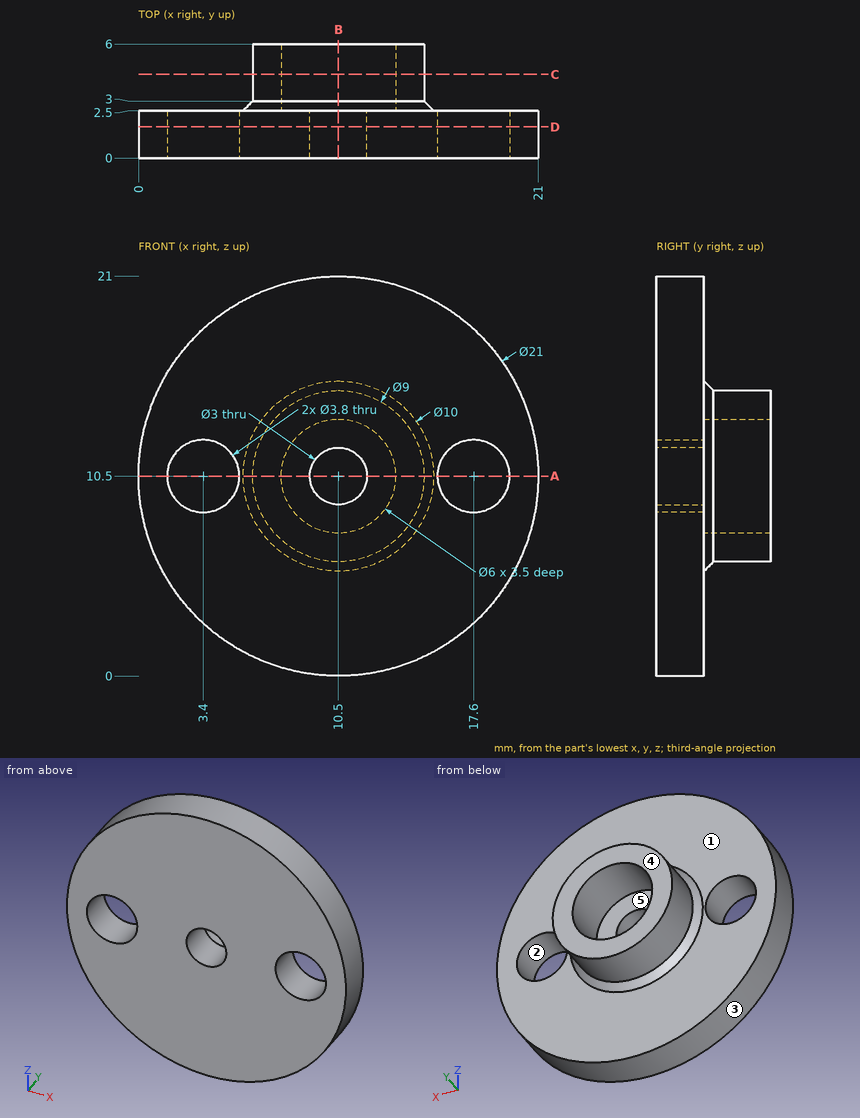
Verification items for this drawing (mm, ordinates from the low corner). A direction names the side the tool comes from. Round coordinates to 2 decimals unless told otherwise and drop trailing zeros. Loops run counter-clockwise (first coordinate to the right, second up) from the corner with the lowest first, then second, coordinate; pieces in that order, holes last. Notation, with made-up numbers: (80.25, 88) - (89.25, 88) arc R24 cw to (89.25, 102) - close; hole circle Ø5 at (-36.75, 2.25). An arc over 180 degrees is marked (long way). Write item = value, one per line.
Q1. Sectioned sample at D-D on y = 1.65. Record the boundary of the cut face in (x, z), plus the area to 3 significant figures.
Here are the results:
outline = circle Ø21 at (10.5, 10.5); hole circle Ø3.8 at (3.4, 10.5); hole circle Ø3 at (10.5, 10.5); hole circle Ø3.8 at (17.6, 10.5)
area = 317 mm^2
Q2. Depth check by flat-ended pin: pin 1 (3 mm diameter, centred on x = 17.6, z = 10.5, fed in from +Y); pin 2 (1.8 mm diameter, centred on x = 10, z = 12, fed in from +Y); pin 3 (1 mm diameter, centred on y = 5, z = 6, fed in from -X); pin 4 (1.5 mm diameter, centred on y = 2.5, z = 12, fed in from +X). Enter the tip coordinate at first touch or a pass-through.
Here are the results:
pin_1 = through
pin_2 = 2.5
pin_3 = 8.44
pin_4 = 20.97
Q3. Sectioned sample at B-B on x = 10.5. Record the boundary of the cut face in (y, z).
Here are the results:
outline = (0, 0) - (2.5, 0) - (2.5, 5.5) - (3, 6) - (6, 6) - (6, 7.5) - (2.5, 7.5) - (2.5, 9) - (0, 9) - close; (0, 12) - (2.5, 12) - (2.5, 13.5) - (6, 13.5) - (6, 15) - (3, 15) - (2.5, 15.5) - (2.5, 21) - (0, 21) - close
Q4. Mould release check, pull along Z, two halves, no side actions. Record for the marked faces 1, 2 and 3: +Z half, -Z half, draft (parallel to the pull), parting line (faces both ways), or undercut.
Here are the results:
face_1 = draft
face_2 = undercut
face_3 = parting line
Q5. Tool access check on the marked faces 4 and 5. Record the directions out of +Z, -Z, +X, -X, +Y, -Y that give a thin tool (end or side, any length) a straight path to the whole face; none if there is none.
Here are the results:
face_4 = +Z, -Z, +X, -X, +Y
face_5 = +Y
Q6. Sectioned sample at A-A on z = 10.5. Record the boundary of the cut face in (x, y).
Here are the results:
outline = (0, 0) - (1.5, 0) - (1.5, 2.5) - (0, 2.5) - close; (5.3, 0) - (9, 0) - (9, 2.5) - (7.5, 2.5) - (7.5, 6) - (6, 6) - (6, 3) - (5.5, 2.5) - (5.3, 2.5) - close; (12, 0) - (15.7, 0) - (15.7, 2.5) - (15.5, 2.5) - (15, 3) - (15, 6) - (13.5, 6) - (13.5, 2.5) - (12, 2.5) - close; (19.5, 0) - (21, 0) - (21, 2.5) - (19.5, 2.5) - close
Q7. Material ranges on L1, parallel to X at y = 0.5, z = 10.5; L2, parallel to Y at x = 5.5, z = 12.25; L3, parallel to Z at x = 10.75, y = 3.25, recorded low to high.
Here are the results:
L1 = 0 to 1.5, 5.3 to 9, 12 to 15.7, 19.5 to 21
L2 = 0 to 2.5
L3 = 6.01 to 7.51, 13.49 to 14.99
Q8. Sectioned sample at C-C on y = 4.4. Record the boundary of the cut face in (x, z).
Here are the results:
outline = circle Ø9 at (10.5, 10.5); hole circle Ø6 at (10.5, 10.5)
